from build123d import *

# Parameters (mm, degrees)
F1_DEPTH = 6.35
F2_R     = 0.50799
F3_F1_R  = 3.175
F3_F2_R  = 3.175
F3_F3_R  = 3.175
F3_F4_R  = 3.175
F3_F5_R  = 3.175
F3_F6_R  = 3.175
F3_F7_R  = 3.1746
F3_F8_R  = 3.1746
F4_R     = 7.62
F5_DEPTH = 2.54


# Not quite as in the source:
# - a fillet or chamfer is up to 0.001 mm smaller than in the source, because OpenCascade refuses the exact size


with BuildPart() as f1:
    # F0 (on Top) → F1 (new body)
    with BuildSketch(Plane.XY):
        Polygon((0, 7.7513456765), (0, 45.3433456765), (-20.32, 45.3433456765), (-20.32, 7.7513456765), (-21.336, 7.7513456765), (-21.336, 6.7353456765), (-20.32, 6.7353456765), (-20.32, -30.8566543235), (0, -30.8566543235), (0, 6.7353456765), (1.016, 6.7353456765), (1.016, 7.7513456765), align=None)
    extrude(amount=F1_DEPTH)

    # F2 (radius 0.508 in the source; OpenCascade refuses exactly that, so slightly less here)
    f2_edges = [f1.edges().sort_by_distance(p)[0] for p in [
        (1.016, 6.735346, 3.175),
        (1.016, 7.751346, 3.175),
        (1.016, 7.243346, 0),
        (1.016, 7.243346, 6.35),
        (0.508, 7.751346, 6.35),
        (0.508, 6.735346, 6.35),
        (0.508, 6.735346, 0),
        (0.508, 7.751346, 0),
        (-21.336, 7.751346, 3.175),
        (-21.336, 6.735346, 3.175),
        (-21.336, 7.243346, 0),
        (-21.336, 7.243346, 6.35),
        (-20.828, 7.751346, 6.35),
        (-20.828, 6.735346, 6.35),
        (-20.828, 7.751346, 0),
        (-20.828, 6.735346, 0),
    ]]
    fillet(f2_edges, radius=F2_R)

    # F3: fillet of radius 3.175 on 16 edges, made by hand

    # F3_f1
    f3_f1_edges = [f1.edges().sort_by_distance(p)[0] for p in [
        (0, -30.8566543235, 3.175),
    ]]
    fillet(f3_f1_edges, radius=F3_F1_R)

    # F3_f2
    f3_f2_edges = [f1.edges().sort_by_distance(p)[0] for p in [
        (-20.32, -30.8566543235, 3.175),
    ]]
    fillet(f3_f2_edges, radius=F3_F2_R)

    # F3_f3
    f3_f3_edges = [f1.edges().sort_by_distance(p)[0] for p in [
        (0, 45.3433456765, 3.175),
    ]]
    fillet(f3_f3_edges, radius=F3_F3_R)

    # F3_f4
    f3_f4_edges = [f1.edges().sort_by_distance(p)[0] for p in [
        (-20.32, 45.3433456765, 3.175),
    ]]
    fillet(f3_f4_edges, radius=F3_F4_R)

    # F3_f5
    f3_f5_edges = [f1.edges().sort_by_distance(p)[0] for p in [
        (-10.16, -30.8566543235, 0),
    ]]
    fillet(f3_f5_edges, radius=F3_F5_R)

    # F3_f6
    f3_f6_edges = [f1.edges().sort_by_distance(p)[0] for p in [
        (-10.16, 45.3433456765, 0),
    ]]
    fillet(f3_f6_edges, radius=F3_F6_R)

    # F3_f7 (radius 3.175 in the source; OpenCascade refuses exactly that, so slightly less here)
    f3_f7_edges = [f1.edges().sort_by_distance(p)[0] for p in [
        (-10.16, 45.3433456765, 6.35),
    ]]
    fillet(f3_f7_edges, radius=F3_F7_R)

    # F3_f8 (radius 3.175 in the source; OpenCascade refuses exactly that, so slightly less here)
    f3_f8_edges = [f1.edges().sort_by_distance(p)[0] for p in [
        (-10.16, -30.8566543235, 6.35),
    ]]
    fillet(f3_f8_edges, radius=F3_F8_R)

    # F4 (on face) → F5 (cut)
    with BuildSketch(Plane(origin=(0, 0, 0), x_dir=(1, 0, 0), z_dir=(0, 0, -1))):
        with Locations((-10.16, -7.2433456765)):
            Circle(F4_R)
    extrude(amount=-F5_DEPTH, mode=Mode.SUBTRACT)


solid = f1.part
Verification items for the finished model (mm, model axes). A direction names the side the tool comes from. Coordinates: 2 decimals unless noted, no trailing zeros. One line per item, written item: value. Start each with the question number.
Item 1: Mould release check, pull along Y, two halves, no side actions. Record for faces 1 (the flat face through (-10, -12, 0)), 2 (the flat face through (-10, 7, 2.54)), 3 (the flat face through (-20.5, 7.751, 3.1)), 4 (the cylindrical face through (-17.773, 6.908, 1.252)): released by +Y, released by -Y, zero draft, split by the parting line, or undercut.
Item 2: Access from +Z, -Z, +X, -X, +Y, -Y to the whole of each face (thin tool, end or side, straight path). Record for faces 5 (the cylindrical face through (-0.95, -10.1, 0.91)), 6 (the cylindrical face through (-0.91, 24.95, 5.4)), 7 (the cylindrical face through (-0.95, 25.07, 0.91)), 8 (the flat face through (0.2, 6.735, 3.1)).
Item 3: Scan lines: probe 1 along X at (y, z) = (8, 1.5); probe 2 along X at (y, z) = (22, 3.25); probe 3 along Z at (x, y) = (-7, 10.5). Record each from-to range of solid material in increasing order.
Item 4: Gauge pin test, flat ends, axial feed: pin 1 (1 mm diameter, centred on x = -19.5, z = 3, fed in from +Y); pin 2 (1 mm diameter, centred on x = -14, z = 4.5, fed in from +Y); pin 3 (1 mm diameter, centred on x = -19.5, z = 3, fed in from -Y). Record the tip position at first contact, or that the pin passes through.
Conclusion:
1. face 1: zero draft
1. face 2: undercut
1. face 3: released by +Y
1. face 4: undercut
2. face 5: -Z, +X, -Y
2. face 6: +Z, +X, +Y
2. face 7: -Z, +X, +Y
2. face 8: +X, -Y
3. probe 1: x = -19.84 to -17.74, -2.58 to -0.48
3. probe 2: x = -20.32 to 0
3. probe 3: z = 2.54 to 6.35
4. pin 1: stops at y = 44.74
4. pin 2: stops at y = 45.23
4. pin 3: stops at y = -30.25
